Here's how the part is built. I have some questions about the finished solid (model axes, mm). Face numbers are marked on the shaded views. Give positions to 0.01 mm unless a question says otherwise; leave off trailing zeros. Write each loop counter-clockwise with the first axis right and the second up, starting at its lowest first coordinate (ties: lowest second). Pieces come first, ordered by that corner, then holes. Notation, with made-up numbers: (35.25, 14.5) -> (52.25, 14.5) arc R13 ccw to (52.25, 21.5) -> close; hole circle Ø1 at (32.25, 25.5). An arc over 180 degrees is marked (long way). Put each result on its own line as item: value. Start each with the question number.
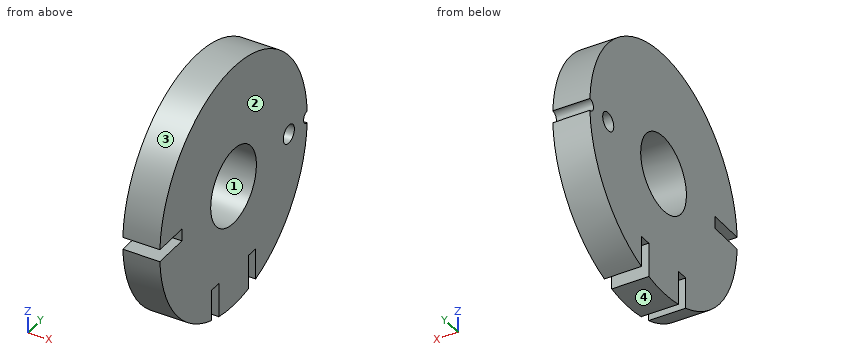
from build123d import *

# Parameters (mm, degrees)
SKETCH1_R           = 10
SKETCH1_R_2         = 3.1
BOSS_EXTRUDE1_DEPTH = 3
SKETCH2_R           = 0.75
SKETCH2_R_2         = 0.5
SKETCH2_W           = 5.709686215
SKETCH2_H           = 1
SKETCH2_W_2         = 1
SKETCH2_H_2         = 4.505813393
CUT_EXTRUDE1_DEPTH  = 3


with BuildPart() as part:
    # Sketch1 → Boss-Extrude1 (new body)
    with BuildSketch(Plane(origin=(0, 0, 0), x_dir=(0, 0, -1), z_dir=(1, 0, 0))):
        Circle(SKETCH1_R)
        Circle(SKETCH1_R_2, mode=Mode.SUBTRACT)
    extrude(amount=BOSS_EXTRUDE1_DEPTH)

    # Sketch2 → Cut-Extrude1 (cut)
    with BuildSketch(Plane(origin=(3, 0, 0), x_dir=(0, 0, -1), z_dir=(1, 0, 0))):
        with Locations((0, 7.5)):
            Circle(SKETCH2_R)
        with Locations((0, 10)):
            Circle(SKETCH2_R_2)
        with Locations((9.854843108, 2.5)):
            Rectangle(SKETCH2_W, SKETCH2_H)
        with Locations((9.854843108, -2.5)):
            Rectangle(SKETCH2_W, SKETCH2_H)
        with Locations((0, -9.252906697)):
            Rectangle(SKETCH2_W_2, SKETCH2_H_2)
    extrude(amount=-CUT_EXTRUDE1_DEPTH, mode=Mode.SUBTRACT)


solid = part.part
1) I want a section at D-D, the plane z = -8. Write out the boundary of the cut face in (x, y).
2) I want a section at B-B, the plane x = 1.85. Write out the boundary of the cut face in (y, z).
3) I need wall thicknesses on probe 1 along Y at (x, z) = (0.9, 1); probe 2 along Z at (x, y) = (0.35, -1.5); probe 3 along Y at (x, z) = (2, 3.75). Which ranges of each line are inside material? Lowest first, please.
4) I want a section at C-C, the plane y = 0. Write out the boundary of the cut face in (x, z).
5) Thinking about a two-plate mould opening in Z: for the marked faces 1, 2, 3 and 4, which applies, released by +Z, released by -Z, zero draft, split by the parting line, or undercut?
6) I want a section at A-A, the plane z = 0. Write out the boundary of the cut face in (x, y), and give its area (3 significant figures).
7) I'm going to push flat-ended pins straight in: pin 1 Ø0.8 at (x, z) = (1.5, -8) entering from -Y; pin 2 Ø6 at (y, z) = (2.5, 7.5) entering from -X; pin 3 Ø0.8 at (x, z) = (1.5, -8) entering from +Y; pin 4 Ø1.5 at (x, y) = (1, 1) entering from -Z. Where does each tip first touch, or does it pass through?
Established:
1. outline: (0, -6) -> (3, -6) -> (3, -3) -> (0, -3) -> close; (0, -2) -> (3, -2) -> (3, 2) -> (0, 2) -> close; (0, 3) -> (3, 3) -> (3, 6) -> (0, 6) -> close
2. outline: (-9.99, -0.5) arc R10 ccw to (-3, -9.54) -> (-3, -7) -> (-2, -7) -> (-2, -9.8) arc R10 ccw to (2, -9.8) -> (2, -7) -> (3, -7) -> (3, -9.54) arc R10 ccw to (9.99, -0.5) arc R0.5 cw to (9.99, 0.5) arc R10 ccw to (-9.99, 0.5) -> (-7, 0.5) -> (-7, -0.5) -> close; hole circle Ø6.2 at (0, 0); hole circle Ø1.5 at (7.5, 0)
3. probe 1: y = -9.95 to -2.93, 2.93 to 9.95
3. probe 2: z = -9.89 to -2.71, 2.71 to 9.89
3. probe 3: y = -9.27 to 9.27
4. outline: (0, -10) -> (3, -10) -> (3, -3.1) -> (0, -3.1) -> close; (0, 3.1) -> (3, 3.1) -> (3, 10) -> (0, 10) -> close
5. face 1: undercut
5. face 2: zero draft
5. face 3: released by +Z
5. face 4: released by -Z
6. outline: (0, -7) -> (3, -7) -> (3, -3.1) -> (0, -3.1) -> close; (0, 3.1) -> (3, 3.1) -> (3, 6.75) -> (0, 6.75) -> close; (0, 8.25) -> (3, 8.25) -> (3, 9.5) -> (0, 9.5) -> close
6. area: 26.4 mm2
7. pin 1: stops at y = -6.5
7. pin 2: stops at x = 0
7. pin 3: stops at y = 6.5
7. pin 4: stops at z = -10
